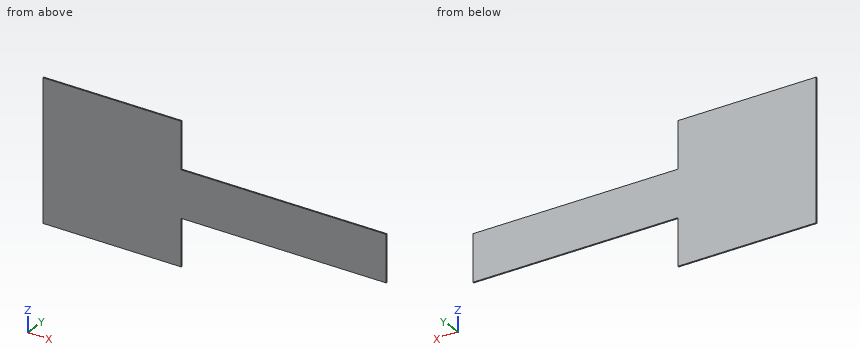
```python
from build123d import *

# Parameters (mm, degrees)
BOSS_EXTRUDE1_DEPTH      = 0.0001
BOSS_EXTRUDE1_DEPTH_BACK = 0.3


with BuildPart() as part:
    # Sketch1 → Boss-Extrude1 (new, two sides: drawn at the far end of the back side and taken through both)
    with BuildSketch(Plane(origin=(0, 0, 0), x_dir=(1, 0, 0), z_dir=(0, 1, 0)).offset(-BOSS_EXTRUDE1_DEPTH_BACK)):
        Polygon((0, -15), (30, -15), (30, -5), (74.5, -5), (74.5, 5), (30, 5), (30, 15), (0, 15), align=None)
    extrude(amount=BOSS_EXTRUDE1_DEPTH + BOSS_EXTRUDE1_DEPTH_BACK)


solid = part.part
```
Read the model definition and answer for the solid it produces. Units are mm, in the model's axes. Give positions to 0.01 mm unless a question says otherwise; leave off trailing zeros. Order: outer loops, then holes, each group sorted by start corner. A loop starts at its lowest first (then second) coordinate and runs counter-clockwise, first axis right, second up. Notation, with made-up numbers: (9.25, 35) -> (53.25, 35) arc R20 ccw to (53.25, 48) -> close; hole circle Ø7 at (85, -38). An arc over 180 degrees is marked (long way). One line per item, written item: value. Start each with the question number.
(1) Straight lines are drawn through the part: L1, parallel to X at y = -0.2, z = -11.75; L2, parallel to Z at x = 41, y = -0.2. For each, find the intervals that lie inside material, in ascending order.
(2) The part is cut by section C-C (x = 69). Determine the outline of the cut face in (y, z).
(3) The part is cut by section A-A (y = -0.2). Determine the outline of the cut face in (x, z), and give its area (4 significant figures).
(4) The part is cut by section B-B (z = 12.75). Determine the outline of the cut face in (x, y).
Taken from the geometry:
1. L1: 0 to 30
1. L2: -5 to 5
2. outline: (-0.3, -5) -> (0, -5) -> (0, 5) -> (-0.3, 5) -> close
3. outline: (0, -15) -> (30, -15) -> (30, -5) -> (74.5, -5) -> (74.5, 5) -> (30, 5) -> (30, 15) -> (0, 15) -> close
3. area: 1,345 mm^2
4. outline: (0, -0.3) -> (30, -0.3) -> (30, 0) -> (0, 0) -> close
